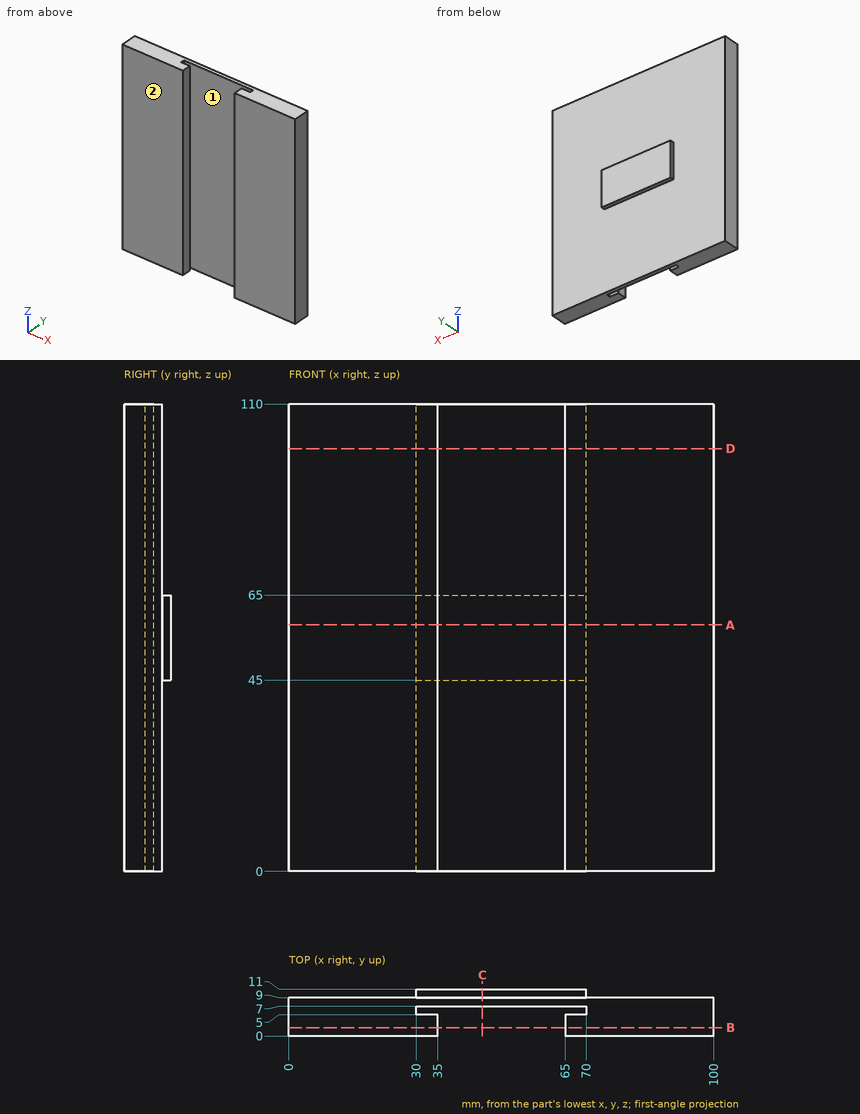
The drawing under review shows one solid part. Ordinate dimensions are in mm from its lowest x, y, z. Coordinates: 2 decimals unless noted, no trailing zeros. Order: outer loops, then holes, each group sorted by start corner. A loop starts at its lowest first (then second) coordinate and runs counter-clockwise, first axis right, second up. Notation, with made-up numbers: (27.25, 3) -> (49.25, 3) arc R23 cw to (49.25, 21) -> close; hole circle Ø1 at (-2, 80). An arc over 180 degrees is marked (long way). Use CSV: the item, a comma, the result in double quotes. Start each with the question number.
Item 1: We need section A-A, the plane z = 58. Give the boundary of the cut face in (x, y), then the cut area to 3 significant figures.
Item 2: Insertion check: pin 1 (0.6 mm diameter, centred on x = 49.5, y = 10, fed in from +Z); pin 2 (10 mm diameter, centred on x = 45, z = 49, fed in from -Y); pin 3 (4 mm diameter, centred on x = 32.5, z = 29.5, fed in from +Y). Each pin has a flat end and moves straight along its axis. Give the tip position at first contact, or say it passes through.
Item 3: We need section C-C, the plane x = 45.5. Give the boundary of the cut face in (y, z), then the cut area to 3 significant figures.
Item 4: We need section D-D, the plane z = 99.5. Give the boundary of the cut face in (x, y), then the cut area to 3 significant figures.
Item 5: Draft analysis for pull direction X (two halves, no side actions). For the marked faces 1 and 2, state which applies: pulls with the +X half, pulls with the -X half, needs draft (parallel to the pull), parting line crosses it, or undercut.
Item 6: Wall thickness on probe 1 along X at (y, z) = (3.5, 64); probe 2 along X at (y, z) = (5.75, 74); probe 3 along X at (y, z) = (10, 62.5): over which ranges is each line inside the solid? List them lowest first.
Item 7: We need section B-B, the plane y = 2. Give the boundary of the cut face in (x, z).
Derived:
1,outline,"(0, 0) -> (35, 0) -> (35, 5) -> (30, 5) -> (30, 7) -> (70, 7) -> (70, 5) -> (65, 5) -> (65, 0) -> (100, 0) -> (100, 9) -> (70, 9) -> (70, 11) -> (30, 11) -> (30, 9) -> (0, 9) -> close"
1,area,"750 mm^2"
2,pin 1,"stops at z = 65"
2,pin 2,"stops at y = 7"
2,pin 3,"stops at y = 9"
3,outline,"(7, 0) -> (9, 0) -> (9, 45) -> (11, 45) -> (11, 65) -> (9, 65) -> (9, 110) -> (7, 110) -> close"
3,area,"260 mm^2"
4,outline,"(0, 0) -> (35, 0) -> (35, 5) -> (30, 5) -> (30, 7) -> (70, 7) -> (70, 5) -> (65, 5) -> (65, 0) -> (100, 0) -> (100, 9) -> (0, 9) -> close"
4,area,"670 mm^2"
5,face 1,"undercut"
5,face 2,"needs draft"
6,probe 1,"x = 0 to 35, 65 to 100"
6,probe 2,"x = 0 to 30, 70 to 100"
6,probe 3,"x = 30 to 70"
7,outline,"(0, 0) -> (35, 0) -> (35, 110) -> (0, 110) -> close; (65, 0) -> (100, 0) -> (100, 110) -> (65, 110) -> close"
